Geometry: see drawing. Coordinates: mm, zero at the bounding-box minimum. A direction names the side the tool comes from. Give positions to 0.01 mm unless a question says otherwise; leave off trailing zeros. Write each loop counter-clockwise with the first axis right and the second up, starting at its lowest first coordinate (ties: lowest second). Pieces come first, ordered by that corner, then holes. Notation, with made-up numbers: (-12, 26.5) - (32, 26.5) arc R28 ccw to (32, 49.5) - close; hole circle Ø10 at (80, 55). An arc over 180 degrees is marked (long way). One line per question, with ' | ' between items. Start each with the question number.
(1) Draft query along X for the marked faces 4, 5, 6 and 7. Return one class per face: +X half, -X half, draft (parallel to the pull), parting line (faces both ways), or undercut.
(2) Pin query (flat end, axial travel): pin 1 (3 mm diameter, centred on y = 5.5, z = 32, fed in from -X); pin 2 (6.5 mm diameter, centred on x = 36, y = 16, fed in from +Z) (3 decimals); pin 3 (3 mm diameter, centred on x = 39.5, y = 7, fed in from -Z) (3 decimals). Return the tip coordinate at first contact, or that it passes through.
(3) Section D-D, the plane x = 37. Return loops of the section in (y, z) (1 decimal).
(4) Ray query, line 1 (Z direction, x = 33, y = 6.5) (1 decimal); line 2 (X direction, y = 7.25, z = 11.5). Return the intervals inside material, ascending. Write a range as [from, to].
(5) Section A-A, the plane x = 25. State how many separate pieces and enclosed holes the cut face has, plus the area to 3 significant figures.
(6) Access query for the marked faces 1, 2 and 3. Directions: +Z, -Z, +X, -X, +Y, -Y. A direction counts if a zero-diameter tool reaches every point of the face in a straight line with its end or side. Return the directions, or none.
(7) Section B-B, the plane z = 155. Return loops of the section in (x, y) (1 decimal).
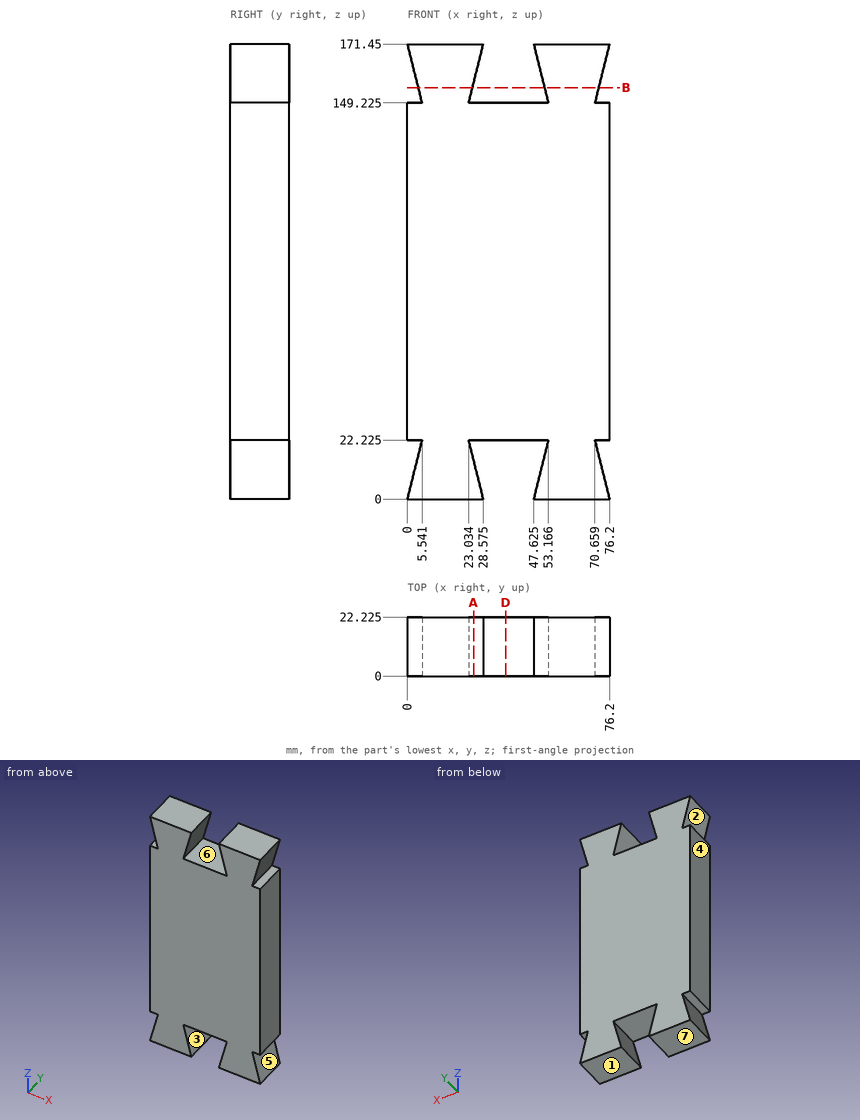
Check sheet entries:
1) face 4: -X half | face 5: +X half | face 6: undercut | face 7: draft
2) pin 1: x = 0 | pin 2: z = 149.225 | pin 3: z = 22.225
3) outline: (0, 22.2) - (22.2, 22.2) - (22.2, 149.2) - (0, 149.2) - close
4) line 1: [22.2, 149.2] | line 2: [2.87, 25.71], [50.49, 73.33]
5) separate pieces: 3 | enclosed holes: 0 | area: 3,460 mm²
6) face 1: -Z, +X, -X, +Y, -Y | face 2: -X, +Y, -Y | face 3: +Y, -Y
7) outline: (4.1, 0) - (24.5, 0) - (24.5, 22.2) - (4.1, 22.2) - close; (51.7, 0) - (72.1, 0) - (72.1, 22.2) - (51.7, 22.2) - close
